Verification items for the finished model (mm, model axes). Give positions to 0.01 mm unless a question says otherwise; leave off trailing zeros. Write each loop counter-clockwise with the first axis right and the second up, starting at its lowest first coordinate (ties: lowest second). Pieces come first, ordered by that corner, then holes. Notation, with made-up numbers: (-0.75, 22) - (33.25, 22) arc R10 cw to (33.25, 39) - close; hole circle Ø8 at (2, 40). An arc over 180 degrees is marked (long way). Put each result on its own line as item: value.
Autodesk Inventor part; units mm, degrees
ref_plane "Work Plane1" through (29, 0, 0) normal (0, -1, 0) x (1, 0, 0)
ref_plane "YZ Plane" through (0, 0, 0) normal (1, 0, 0) x (0, 1, 0)
ref_plane "XZ Plane" through (0, 0, 0) normal (0, 1, 0) x (-1, 0, 0)
sketch "Sketch1" plane through (0, 0, 0) normal (0, 0, 1) x (1, 0, 0)
  line L0 (-2, 0) -> (200, 0)
  line L1 (200, 0) -> (200, 4)
  line L2 (200, 4) -> (172, 4)
  line L3 (172, 4) -> (171.2331, 4)
  line L4 (171.2331, 4) -> (0, 4)
  line L5 (0, 4) -> (0, 6.5)
  line L6 (0, 6.5) -> (-8, 6.5)
  line L7 (-8, 6.5) -> (-8, 3.4641)
  line L8 (-8, 3.4641) -> (-4, 3.4641)
  line L9 (-4, 3.4641) -> (-2, 0)
  line L10 (-41.6, 0) -> (193.6, 0)
  line L11 (0, -1.3) -> (0, 7.8)
  line L12 (172, 4) -> (0, 4) construction
  dimension "d1" = 28
  dimension "d2" = 0.7669
  dimension "d3" = 8
  dimension "d4" = 4
  dimension "d5" = 60
  dimension "d6" = 8
  dimension "d7" = 8
  dimension "d8" = 6.9282
  dimension "d9" = 13
  dimension "d26" = 200
revolve "Body" add sketch "Sketch1" angle 360 about axis through (-2, 0, 0) along (1, 0, 0)
sketch "Sketch2" plane through (-8, 0, 0) normal (-1, 0, 0) x (0, 0, 1)
  circle A0 centre (0, 0) radius 3.4641
  line L0 (0, -9.1) -> (0, 9.1)
  line L1 (-9.1, 0) -> (9.1, 0)
  line L2 (3.4641, 0) -> (1.7321, -3)
  line L3 (1.7321, -3) -> (-1.7321, -3)
  line L4 (-1.7321, -3) -> (-3.4641, 0)
  line L5 (-3.4641, 0) -> (-1.7321, 3)
  line L6 (-1.7321, 3) -> (1.7321, 3)
  line L7 (1.7321, 3) -> (3.4641, 0)
extrude "Slot" add sketch "Sketch2" against normal up to next contours L7 A0 | A0 L2 | L6 L0 A0 | A0 L0 L3 | L0 L6 A0 | A0 L3 L0 | L4 A0 | A0 L5
fillet "Fillet1" radius 0.8 1 edges at (-8, -6.5, 0)
thread "Thread"
chamfer "Chamfer1" distance 0.7668 distance2 0.7668 1 edges at (200, -4, 0) measured on face at (200, -0.5839, -0.3933)
ref_plane "Work Plane1" through (29, 0, 0) normal (0, -1, 0) x (1, 0, 0)
fillet "Fillet2" radius 0.1 1 edges at (0, -4, 0)
equation "\"d1\" = GEL"
equation "\"d3\" = KOH"
equation "\"d4\" = INTI"
equation "\"d6\" = GD"
equation "\"d7\" = BDM"
equation "\"d8\" = 1.1547 * SW"
equation "\"d9\" = KOD"
equation "\"d26\" = NLG"
equation "\"d30\" = R"
equation "\"d17\" = RR"
equation "\"d13\" = GEL"
equation "\"d15\" = -0.5 * SPD + 0.5 * GD"
equation "\"d16\" = GUL"
equation "\"GD\" = NND"
equation "\"NLG\" = 200"
equation "\"GEL\" = 28"
equation "\"KOD\" = 13"
equation "\"KOH\" = 8"
equation "\"INTI\" = 4"
equation "\"GAL\" = 0.61345 * PTC"
equation "\"GUL\" = 0.61345 * PTC"
equation "\"BDM\" = NND"
equation "\"SW\" = 6"
equation "\"RR\" = 0.8"
equation "\"SPD\" = 6.46638"
equation "\"R\" = 0.1"
equation "\"TOA\" = 30deg"
equation "\"THREADDIA\" = 8"
equation "\"PTC\" = 1.25"
equation "\"NND\" = 8"
equation "\"E0\" = 1.155 * SW"
equation "\"GD1\" = THREADDIA - 1.2269 * PTC"
properties part number "ANSI B18.3.1M - M8x1.25 x 160" material "Steel, Mild"
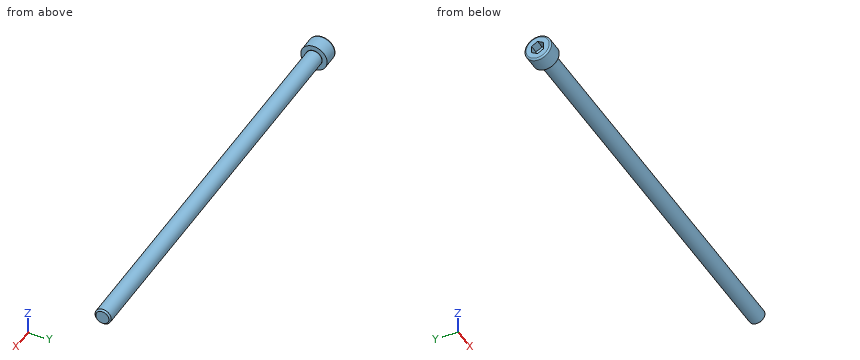
Q1. Go/stop test with flat-tipped pins: pin 1 Ø1 at (y, z) = (-2, -1.5) entering from -X; pin 2 Ø1.5 at (x, z) = (69, -1) entering from -Y; pin 3 Ø1.5 at (y, z) = (-2, 5) entering from +X. Record where each tip stops, or that it passes through.
Answers follow:
pin 1: stops at x = -3.73
pin 2: stops at y = -3.99
pin 3: stops at x = 0
Q2. Scan lines: line 1 along Y through (x, z) = (144, -2); line 2 along Z through (x, y) = (83.5, -0.5); line 3 along X through (y, z) = (4, 4). Record each from-to range of solid material in increasing order.
Answers follow:
line 1: y = -3.46 to 3.46
line 2: z = -3.97 to 3.97
line 3: x = -8 to 0
Q3. Section check A-A, the plane x = 23. Record the cut outline in (y, z), plus the area to 3 significant figures.
Answers follow:
outline: circle Ø8 at (0, 0)
area: 50.3 mm2
